from build123d import *

# Parameters (mm, degrees)
SKETCH1_R           = 5
BOSS_EXTRUDE1_DEPTH = 2
SKETCH2_W           = 96.58456166
SKETCH2_H           = 1.682573812
BOSS_EXTRUDE2_DEPTH = 3.5
FILLET1_R           = 2


with BuildPart() as part:
    # Sketch1 → Boss-Extrude1 (new body)
    with BuildSketch(Plane.XY):
        with BuildLine():
            Line((-58.7, 0), (58.7, 0))
            ThreePointArc((58.7, 0), (69.7, 11), (58.7, 22))
            Line((58.7, 22), (-58.7, 22))
            ThreePointArc((-58.7, 22), (-69.7, 11), (-58.7, 0))
        make_face()
        with Locations((-58.7, 11)):
            Circle(SKETCH1_R, mode=Mode.SUBTRACT)
        with Locations((58.7, 11)):
            Circle(SKETCH1_R, mode=Mode.SUBTRACT)
    extrude(amount=BOSS_EXTRUDE1_DEPTH)

    # Sketch2 → Boss-Extrude2 (add)
    with BuildSketch(Plane.XY.offset(2)):
        with Locations((-0.304491052, 21.158713094)):
            Rectangle(SKETCH2_W, SKETCH2_H)
    boss_extrude2 = extrude(amount=BOSS_EXTRUDE2_DEPTH)

    # Mirror1: Boss-Extrude2 across plane
    add(boss_extrude2.mirror(Plane.XY.offset(5.5)))

    # Mirror2: part across plane


with BuildPart() as part_1:
    add(part.part)
    add(part.part.mirror(Plane(origin=(0, 0, 9), x_dir=(1, 0, 0), z_dir=(0, 0, -1))))

    # Fillet1
    fillet1_edges = [part_1.edges().sort_by_distance(p)[0] for p in [
        (-48.596771882, 21.158713094, 2),
        (47.987789778, 21.158713094, 2),
        (-48.596771882, 21.158713094, 16),
        (47.987789778, 21.158713094, 16),
    ]]
    fillet(fillet1_edges, radius=FILLET1_R)


solid = part_1.part
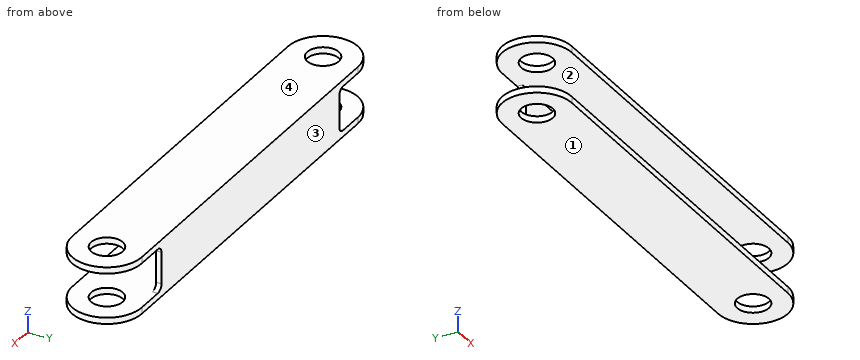
Geometry check sheet. Reference: the model listing, model coordinates, mm. Face numbers are marked on the shaded views. Give positions to 0.01 mm unless a question says otherwise; leave off trailing zeros. Order: outer loops, then holes, each group sorted by start corner. A loop starts at its lowest first (then second) coordinate and runs counter-clockwise, first axis right, second up. Notation, with made-up numbers: (-13.5, 65.25) - (27.5, 65.25) arc R30 cw to (27.5, 98.25) - close; hole circle Ø8 at (58.25, -9.75). An arc over 180 degrees is marked (long way). Use one line per item in the form item = value.
1) Sectioned sample at C-C (y = 2). Record the boundary of the cut face in (x, z).
Working result:
outline = (-65.02, 0) - (65.02, 0) - (65.02, 2) - (-65.02, 2) - close; (-65.02, 16) - (65.02, 16) - (65.02, 18) - (-65.02, 18) - close
2) Sectioned sample at B-B (x = 57.5). Record the boundary of the cut face in (y, z), and give its area (3 significant figures).
Working result:
outline = (0, 0) - (6.15, 0) - (6.15, 2) - (0, 2) - close; (0, 16) - (6.15, 16) - (6.15, 18) - (0, 18) - close; (15.85, 0) - (22, 0) - (22, 2) - (15.85, 2) - close; (15.85, 16) - (22, 16) - (22, 18) - (15.85, 18) - close
area = 49.2 mm^2
3) Depth check by flat-ended pin: pin 1 Ø12 at (x, y) = (-19, 6.5) entering from -Z; pin 2 Ø7 at (x, z) = (-15.5, 9) entering from -Y; pin 3 Ø1.3 at (y, z) = (21.5, 6.5) entering from -X; pin 4 Ø1.9 at (y, z) = (21, 7) entering from +X. Enter the tip coordinate at first touch or a pass-through.
Working result:
pin_1 = 0
pin_2 = 20.32
pin_3 = -48.6
pin_4 = 47.99
4) Sectioned sample at D-D (x = 11). Record the boundary of the cut face in (y, z).
Working result:
outline = (0, 0) - (22, 0) - (22, 18) - (0, 18) - (0, 16) - (20.32, 16) - (20.32, 2) - (0, 2) - close
5) Material ranges on probe 1 along Z at (x, y) = (14, 4.5); probe 2 along Y at (x, z) = (-58.7, 16.8); probe 3 along Y at (x, z) = (39.5, 4.75), recorded low to high. Write a range as from..to.
Working result:
probe_1 = 0..2, 16..18
probe_2 = 0..6, 16..22
probe_3 = 20.32..22
6) Draft check along Z on the marked faces 1, 2, 3 and 4. Enter one of: released by +Z, released by -Z, zero draft, split by the parting line, or undercut.
Working result:
face_1 = released by -Z
face_2 = undercut
face_3 = zero draft
face_4 = released by +Z
7) Sectioned sample at A-A (y = 11). Record the boundary of the cut face in (x, z).
Working result:
outline = (-69.7, 0) - (-63.7, 0) - (-63.7, 2) - (-69.7, 2) - close; (-69.7, 16) - (-63.7, 16) - (-63.7, 18) - (-69.7, 18) - close; (-53.7, 0) - (53.7, 0) - (53.7, 2) - (-53.7, 2) - close; (-53.7, 16) - (53.7, 16) - (53.7, 18) - (-53.7, 18) - close; (63.7, 0) - (69.7, 0) - (69.7, 2) - (63.7, 2) - close; (63.7, 16) - (69.7, 16) - (69.7, 18) - (63.7, 18) - close
